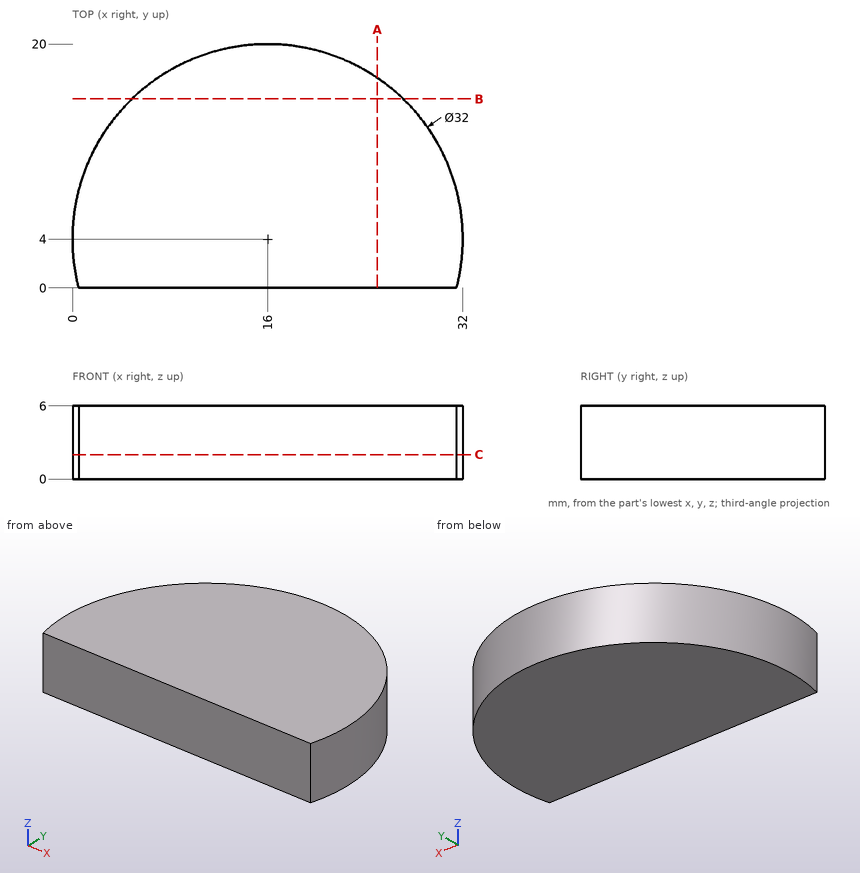
Here's the drawing with two shaded views (mm, measured from the low corner). I have some questions. Round coordinates to 2 decimals unless told otherwise and drop trailing zeros. Loops run counter-clockwise (first coordinate to the right, second up) from the corner with the lowest first, then second, coordinate; pieces in that order, holes last. Notation, with made-up numbers: (78, 51.5) - (115, 51.5) arc R24 cw to (115, 62.5) - close; hole circle Ø7 at (52, 14). An arc over 180 degrees is marked (long way). Write item = value, one per line.
1) Imagine slicing it at A-A (x = 25). Please give me the cut outline in (y, z), and give its area (3 significant figures).
Computed:
outline = (0, 0) - (17.23, 0) - (17.23, 6) - (0, 6) - close
area = 103 mm2
2) I'm going to push flat-ended pins straight in: P1, Ø1, axis at y = 11.5, z = 4, coming from the +X side; P2, Ø2, axis at x = 5.5, z = 3, coming from the +Y side; P3, Ø12, axis at x = 9, y = 17, coming from the -Z side. Where does each tip first touch, or does it pass through?
Computed:
P1 = 30.39
P2 = 16.87
P3 = 0
3) Imagine slicing it at C-C (z = 2). Please give me the cut outline in (x, y).
Computed:
outline = (0.51, 0) - (31.49, 0) arc R16 ccw (long way) to start
4) Imagine slicing it at B-B (y = 15.5). Please give me the cut outline in (x, z), and give its area (3 significant figures).
Computed:
outline = (4.88, 0) - (27.12, 0) - (27.12, 6) - (4.88, 6) - close
area = 133 mm2
5) I need wall thicknesses on line 1 along X through (y, z) = (3.75, 0.55); line 2 along Y through (x, z) = (17, 1.9); line 3 along Y through (x, z) = (21.5, 3.95). Which ranges of each line are inside material? Lowest first, please. Write a range as from..to.
Computed:
line_1 = 0..32
line_2 = 0..19.97
line_3 = 0..19.02
